Geometry check sheet. Reference: the model listing, model coordinates, mm. A direction names the side the tool comes from. Round coordinates to 2 decimals unless told otherwise and drop trailing zeros. Loops run counter-clockwise (first coordinate to the right, second up) from the corner with the lowest first, then second, coordinate; pieces in that order, holes last. Notation, with made-up numbers: (57.25, 1.25) - (103.25, 1.25) arc R23 ccw to (103.25, 31.25) - close; hole circle Ø10 at (-32, 51). An arc over 180 degrees is marked (long way). Write item = value, one per line.
```python
from build123d import *

# Parameters (mm, degrees)
SKETCH1_W           = 165.1
SKETCH1_H           = 85.09
BOSS_EXTRUDE2_DEPTH = 12.7
SKETCH3_W           = 139.7
SKETCH3_H           = 85.09
BOSS_EXTRUDE3_DEPTH = 38.1
SKETCH4_W           = 120.65
SKETCH4_H           = 66.04
CUT_EXTRUDE1_DEPTH  = 44.45
SKETCH5_R           = 1.5875
CUT_EXTRUDE3_DEPTH  = 154.98717268
SKETCH8_R           = 1.5875
CUT_EXTRUDE4_DEPTH  = 25.4
SKETCH11_R          = 1.5875
CUT_EXTRUDE6_DEPTH  = 153.275595057
CUT_EXTRUDE7_DEPTH  = 3.175
CUT_EXTRUDE8_REACH  = 176.92
SKETCH15_W          = 25.4
SKETCH15_H          = 19.05


with BuildPart() as part:
    # Sketch1 → Boss-Extrude2 (new body)
    with BuildSketch(Plane(origin=(0, 0, 0), x_dir=(1, 0, 0), z_dir=(0, 1, 0))):
        with Locations((47.625, 26.67)):
            Rectangle(SKETCH1_W, SKETCH1_H)
    extrude(amount=BOSS_EXTRUDE2_DEPTH)

    # Sketch3 → Boss-Extrude3 (add)
    with BuildSketch(Plane(origin=(0, 12.7, 0), x_dir=(1, 0, 0), z_dir=(0, 1, 0))):
        with Locations((47.625, 26.67)):
            Rectangle(SKETCH3_W, SKETCH3_H)
    extrude(amount=BOSS_EXTRUDE3_DEPTH)

    # Sketch4 → Cut-Extrude1 (cut)
    with BuildSketch(Plane(origin=(0, 50.8, 0), x_dir=(1, 0, 0), z_dir=(0, 1, 0))):
        with Locations((47.625, 26.67)):
            Rectangle(SKETCH4_W, SKETCH4_H)
    extrude(amount=-CUT_EXTRUDE1_DEPTH, mode=Mode.SUBTRACT)

    # Sketch5 → Cut-Extrude3 (cut, through all)
    with BuildSketch(Plane(origin=(0, 6.35, 0), x_dir=(1, 0, 0), z_dir=(0, 1, 0))):
        with Locations(Location((15.24, 50.8, 0), (0, 0, 270))):
            Circle(SKETCH5_R)
        with Locations(Location((13.97, 2.54, 0), (0, 0, 270))):
            Circle(SKETCH5_R)
        with Locations(Location((90.17, 50.8, 0), (0, 0, 270))):
            Circle(SKETCH5_R)
        with Locations(Location((96.52, 2.54, 0), (0, 0, 270))):
            Circle(SKETCH5_R)
    extrude(amount=-CUT_EXTRUDE3_DEPTH, mode=Mode.SUBTRACT)

    # Sketch8 → Cut-Extrude4 (cut)
    with BuildSketch(Plane(origin=(0, 50.8, 0), x_dir=(1, 0, 0), z_dir=(0, 1, 0))):
        with Locations(Location((-17.4625, 64.4525, 0), (0, 0, 270))):
            Circle(SKETCH8_R)
        with Locations(Location((-17.4625, -11.1125, 0), (0, 0, 270))):
            Circle(SKETCH8_R)
        with Locations(Location((112.7125, -11.1125, 0), (0, 0, 270))):
            Circle(SKETCH8_R)
        with Locations(Location((112.7125, 64.4525, 0), (0, 0, 270))):
            Circle(SKETCH8_R)
    extrude(amount=-CUT_EXTRUDE4_DEPTH, mode=Mode.SUBTRACT)

    # Sketch11 → Cut-Extrude6 (cut, through all)
    with BuildSketch(Plane(origin=(0, 12.7, 0), x_dir=(1, 0, 0), z_dir=(0, 1, 0))):
        with Locations(Location((-28.575, 62.865, 0), (0, 0, 270))):
            Circle(SKETCH11_R)
        with Locations(Location((-28.575, -9.525, 0), (0, 0, 270))):
            Circle(SKETCH11_R)
        with Locations(Location((123.825, -9.525, 0), (0, 0, 270))):
            Circle(SKETCH11_R)
        with Locations(Location((123.825, 62.865, 0), (0, 0, 270))):
            Circle(SKETCH11_R)
    extrude(amount=-CUT_EXTRUDE6_DEPTH, mode=Mode.SUBTRACT)

    # Sketch14 → Cut-Extrude7 (cut)
    with BuildSketch(Plane.XZ):
        Polygon((17.057033947, -1.79780972), (14.870761336, 0.50454496), (11.783727389, -0.23764532), (10.882966053, -3.28219028), (13.069238664, -5.58454496), (16.156272611, -4.84235468), align=None)
        Polygon((18.415, -50.8), (16.8275, -48.050369343), (13.6525, -48.050369343), (12.065, -50.8), (13.6525, -53.549630657), (16.8275, -53.549630657), align=None)
        Polygon((93.009008497, -52.221497715), (92.820557381, -49.052095378), (89.981548884, -47.630597662), (87.330991503, -49.378502285), (87.519442619, -52.547904622), (90.358451116, -53.969402338), align=None)
        Polygon((99.581036114, -3.383020112), (98.78059489, -0.310575019), (95.719558776, 0.532445092), (93.458963886, -1.696979888), (94.25940511, -4.769424981), (97.320441224, -5.612445092), align=None)
    extrude(amount=-CUT_EXTRUDE7_DEPTH, mode=Mode.SUBTRACT)

    # Sketch15 → Cut-Extrude8 (cut, up to next)
    with BuildSketch(Plane.ZY.offset(22.225), mode=Mode.PRIVATE) as cut_extrude8_sk1:
        with Locations((-31.115, 28.575)):
            Rectangle(SKETCH15_W, SKETCH15_H)
    cut_extrude8_tool1 = extrude(cut_extrude8_sk1.sketch, amount=-CUT_EXTRUDE8_REACH, mode=Mode.PRIVATE) & part.part
    add(cut_extrude8_tool1.solids().sort_by_distance((-22.225, 28.575, -31.115))[0], mode=Mode.SUBTRACT)


solid = part.part
```
(1) Gauge pin test, flat ends, axial feed: pin 1 (2.5 mm diameter, centred on x = 14.5, z = -50, fed in from -Y) (3 decimals); pin 2 (2 mm diameter, centred on y = 32, z = -27.5, fed in from +X) (3 decimals); pin 3 (4 mm diameter, centred on x = 96.52, z = -2.54, fed in from +Y). Record the tip position at first contact, or that the pin passes through.
Answers follow:
pin_1 = 3.175
pin_2 = 117.475
pin_3 = 6.35
(2) Set-up check for faces 4 (the flat face through (87.424, 1.565, -50.941)), 5 (the cylindrical face through (114.286, 38.278, 10.906)), 6 (the flat face through (-18, 28, -18.415)): record each of +Z, -Z, +X, -X, +Y, -Y from which the full face is reachable in a straight line by a thin tool's end or side.
Answers follow:
face_4 = -Y
face_5 = +Y
face_6 = -X
(3) Section check B-B (x = 30.5). Enter the section's corners in (y, z) (3 decimals).
Answers follow:
outline = (0, -69.215) - (50.8, -69.215) - (50.8, -59.69) - (6.35, -59.69) - (6.35, 6.35) - (50.8, 6.35) - (50.8, 15.875) - (0, 15.875) - close
(4) Section check A-A (y = 15.5). Enter the section's corners in (x, z) (3 decimals).
Answers follow:
outline = (-22.225, -69.215) - (117.475, -69.215) - (117.475, 15.875) - (-22.225, 15.875) - close; hole (-12.7, -59.69) - (107.95, -59.69) - (107.95, 6.35) - (-12.7, 6.35) - close
(5) Mould release check, pull along Z, two halves, no side actions. Record for faces 1 (the flat face through (46, 25, 15.875)), 2 (the cylindrical face through (88.62, 4.78, -51.14)), 3 (the flat face through (-22.225, 40, -26)): pulls with the +Z half, pulls with the -Z half, needs draft (parallel to the pull), parting line crosses it, or undercut.
Answers follow:
face_1 = pulls with the +Z half
face_2 = undercut
face_3 = needs draft
(6) Section check C-C (y = 30.5). State how many separate pieces and enclosed holes the cut face has, then the cut area to 3 significant figures.
Answers follow:
separate_pieces = 1
enclosed_holes = 4
area = 3,650 mm²
(7) Section check D-D (z = -13). Enter the section's corners in (x, y) (3 decimals), then the cut area to 3 significant figures.
Answers follow:
outline = (-34.925, 0) - (130.175, 0) - (130.175, 12.7) - (117.475, 12.7) - (117.475, 50.8) - (107.95, 50.8) - (107.95, 6.35) - (-12.7, 6.35) - (-12.7, 50.8) - (-22.225, 50.8) - (-22.225, 12.7) - (-34.925, 12.7) - close
area = 2,060 mm²
(8) Scan lines: L1, parallel to X at y = 5.5, z = -50.8 (1 decimal); L2, parallel to Z at x = 74.5, y = 34 (3 decimals); L3, parallel to X at y = 47.5, z = -54.5 (3 decimals). Record each from-to range of solid material in increasing order. Write a range as [from, to].
Answers follow:
L1 = [-34.9, 13.7], [16.8, 88.6], [91.8, 130.2]
L2 = [-69.215, -59.69], [6.35, 15.875]
L3 = [-22.225, -12.7], [107.95, 117.475]
